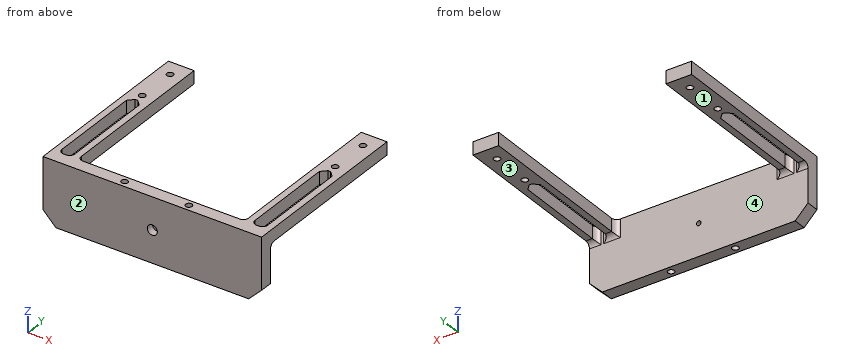
from build123d import *

# Parameters (mm, degrees)
SKETCH1_R           = 1.25
BOSS_EXTRUDE1_DEPTH = 5
SKETCH2_W           = 85
SKETCH2_H           = 5
BOSS_EXTRUDE2_DEPTH = 20
FILLET1_R           = 2
CUT_EXTRUDE1_DEPTH  = 25
SKETCH9_R           = 1.25
CUT_EXTRUDE2_DEPTH  = 58
SKETCH10_R          = 1.95
CUT_EXTRUDE3_DEPTH  = 2.9
SKETCH11_R          = 0.9
CUT_EXTRUDE4_DEPTH  = 6.9
CHAMFER1_SIZE       = 5


with BuildPart() as part:
    # Sketch1 → Boss-Extrude1 (new body)
    with BuildSketch(Plane.XY):
        Polygon((-32.5, 0), (32.5, 0), (32.5, 65), (42.5, 65), (42.5, 0), (42.5, -5), (-42.5, -5), (-42.5, 0), (-42.5, 65), (-32.5, 65), align=None)
        with Locations((37.5, 58.75)):
            Circle(SKETCH1_R, mode=Mode.SUBTRACT)
        with Locations((37.5, 43.25)):
            Circle(SKETCH1_R, mode=Mode.SUBTRACT)
        with Locations(Location((-37.5, 58.75, 0), (0, 0, 180))):
            Circle(SKETCH1_R, mode=Mode.SUBTRACT)
        with Locations(Location((-37.5, 43.25, 0), (0, 0, 180))):
            Circle(SKETCH1_R, mode=Mode.SUBTRACT)
    extrude(amount=BOSS_EXTRUDE1_DEPTH)

    # Sketch2 → Boss-Extrude2 (add)
    with BuildSketch(Plane(origin=(0, 0, 0), x_dir=(-1, 0, 0), z_dir=(0, 0, -1))):
        with Locations((0, -2.5)):
            Rectangle(SKETCH2_W, SKETCH2_H)
    extrude(amount=BOSS_EXTRUDE2_DEPTH)

    # Fillet1
    fillet1_edges = [part.edges().sort_by_distance(p)[0] for p in [
        (-37.5, 0, 0),
        (-32.5, 0, 2.5),
        (32.5, 0, 2.5),
        (37.5, 0, 0),
    ]]
    fillet(fillet1_edges, radius=FILLET1_R)

    # Sketch8 → Cut-Extrude1 (cut)
    with BuildSketch(Plane.XY.offset(5)):
        with BuildLine():
            Line((-38, 0), (-37, 0))
            ThreePointArc((-37, 0), (-35.585786438, 0.585786438), (-35, 2))
            Line((-35, 2), (-35, 38))
            Line((-35, 38), (-37, 40))
            Line((-37, 40), (-38, 40))
            Line((-38, 40), (-40, 38))
            Line((-40, 38), (-40, 2))
            ThreePointArc((-40, 2), (-39.414213562, 0.585786438), (-38, 0))
        make_face()
        with BuildLine():
            Line((38, 0), (37, 0))
            ThreePointArc((37, 0), (35.585786438, 0.585786438), (35, 2))
            Line((35, 2), (35, 38))
            Line((35, 38), (37, 40))
            Line((37, 40), (38, 40))
            Line((38, 40), (40, 38))
            Line((40, 38), (40, 2))
            ThreePointArc((40, 2), (39.414213562, 0.585786438), (38, 0))
        make_face()
    extrude(amount=-CUT_EXTRUDE1_DEPTH, mode=Mode.SUBTRACT)

    # Sketch9 → Cut-Extrude2 (cut)
    with BuildSketch(Plane(origin=(0, 0, -20), x_dir=(-1, 0, 0), z_dir=(0, 0, -1))):
        with Locations((12.5, -2.5)):
            Circle(SKETCH9_R)
        with Locations((-12.5, -2.5)):
            Circle(SKETCH9_R)
    extrude(amount=-CUT_EXTRUDE2_DEPTH, mode=Mode.SUBTRACT)

    # Sketch10 → Cut-Extrude3 (cut)
    with BuildSketch(Plane.XZ.offset(5)):
        with Locations(Location((0, -7.5, 0), (0, 0, 270))):
            Circle(SKETCH10_R)
    extrude(amount=-CUT_EXTRUDE3_DEPTH, mode=Mode.SUBTRACT)

    # Sketch11 → Cut-Extrude4 (cut)
    with BuildSketch(Plane.XZ.offset(2.1)):
        with Locations(Location((0, -7.5, 0), (0, 0, 270))):
            Circle(SKETCH11_R)
    extrude(amount=-CUT_EXTRUDE4_DEPTH, mode=Mode.SUBTRACT)

    # Chamfer1
    chamfer1_edges = [part.edges().sort_by_distance(p)[0] for p in [
        (-42.5, -2.5, -20),
        (42.5, -2.5, -20),
    ]]
    chamfer(chamfer1_edges, length=CHAMFER1_SIZE)


solid = part.part
CAD build for the part. Positions are in the model's coordinates, mm. Face numbers are marked on the shaded views. A direction names the side the tool comes from. Round coordinates to 2 decimals unless told otherwise and drop trailing zeros. Write each loop counter-clockwise with the first axis right and the second up, starting at its lowest first coordinate (ties: lowest second). Pieces come first, ordered by that corner, then holes. Notation, with made-up numbers: (-5, -37) -> (10, -37) arc R25 cw to (10, -8) -> close; hole circle Ø4 at (-26.5, 76). An arc over 180 degrees is marked (long way). Answer as a JSON object with one key per item and string values.
(1) Band-saw the part on A-A, the plane y = 5. List the corners of the cut face in (x, z).
Reported:
{"outline": "(-42.5, 0) -> (-40, 0) -> (-40, 5) -> (-42.5, 5) -> close; (-35, 0) -> (-32.5, 0) -> (-32.5, 5) -> (-35, 5) -> close; (32.5, 0) -> (35, 0) -> (35, 5) -> (32.5, 5) -> close; (40, 0) -> (42.5, 0) -> (42.5, 5) -> (40, 5) -> close"}
(2) Band-saw the part on B-B, the plane x = -12.5. List the corners of the cut face in (y, z).
Reported:
{"outline": "(-5, -20) -> (-3.75, -20) -> (-3.75, 5) -> (-5, 5) -> close; (-1.25, -20) -> (0, -20) -> (0, 5) -> (-1.25, 5) -> close"}
(3) Probe probe 1 along X at (y, z) = (2.5, 3.5); probe 2 along Y at (x, z) = (37.5, 3.05); probe 3 along Y at (x, z) = (12.5, -14.75). List the from-to ranges inside material, lowest first. Write a range as [from, to].
Reported:
{"probe 1": "x = [-42.5, -40], [-35, -32.5], [32.5, 35], [40, 42.5]", "probe 2": "y = [-5, 0], [40, 42], [44.5, 57.5], [60, 65]", "probe 3": "y = [-5, -3.75], [-1.25, 0]"}
(4) Which spindle directions (+Z, -Z, +X, -X, +Y, -Y) get a long thin tool onto all of the face, cutting with end or side? Do the marked faces 1 and 2. Say none if no direction does.
Reported:
{"face 1": "-Z, +X, -X, +Y", "face 2": "+Z, -Z, +X, -X, -Y"}
(5) Band-saw the part on D-D, the plane z = -12.75. List the corners of the cut face in (x, y).
Reported:
{"outline": "(-42.5, -5) -> (42.5, -5) -> (42.5, 0) -> (-42.5, 0) -> close; hole circle Ø2.5 at (-12.5, -2.5); hole circle Ø2.5 at (12.5, -2.5)"}
(6) Two-plate mould, pull along X, no slides. Class the marked faces 3 and 4: +X half, -X half, draft (parallel to the pull), parting line (faces both ways), or undercut.
Reported:
{"face 3": "draft", "face 4": "undercut"}
(7) Pin check, flat tips, straight feed: P1, Ø2, axis at x = 0, z = -7.5, coming from the -Y side; P2, Ø1, axis at x = -4, z = -11.5, coming from the +Y side; P3, Ø4, axis at x = -12.5, y = -2.5, coming from the +Z side. Stop position of each tip, or through.
Reported:
{"P1": "stops at y = -2.1", "P2": "stops at y = 0", "P3": "stops at z = 5"}
(8) Band-saw the part on C-C, the plane y = 52. List the corners of the cut face in (x, z), then the cut area to 3 significant figures.
Reported:
{"outline": "(-42.5, 0) -> (-32.5, 0) -> (-32.5, 5) -> (-42.5, 5) -> close; (32.5, 0) -> (42.5, 0) -> (42.5, 5) -> (32.5, 5) -> close", "area": "100 mm^2"}
